```python
from build123d import *

# Parameters (mm, degrees)
F0_R     = 25.4
F0_R_2   = 15.875
F1_DEPTH = 8.89
F3_R     = 3.175
F4_REACH = 59.7812561211
F6_R     = 3.175
F7_REACH = 59.7812562211
F8_SIZE  = 0.762
F9_SIZE  = 0.762


with BuildPart() as f1:
    # F0 (on Right) → F1 (new body)
    with BuildSketch(Plane.YZ):
        Circle(F0_R)
        Circle(F0_R_2, mode=Mode.SUBTRACT)
    extrude(amount=F1_DEPTH)

    f4_end = f1.faces().sort_by_distance((4.445, -15.875, 0))[0]
    # F3 (on offset) → F4 (cut, up to a face of the model that its end follows)
    with BuildSketch(Plane.XZ.offset(25.4)):
        with Locations((4.064, 0)):
            Circle(F3_R)
    f4_long = extrude(amount=-F4_REACH, mode=Mode.PRIVATE)
    add(split(f4_long, bisect_by=f4_end, keep=Keep.ALL, mode=Mode.PRIVATE).solids().sort_by_distance((4.064, -25.4, 0))[0], mode=Mode.SUBTRACT)

    f7_end = f1.faces().sort_by_distance((0.457728864, -15.875, 0))[0]
    # F6 (on offset) → F7 (cut, up to a face of the model that its end follows)
    with BuildSketch(Plane.XY.offset(25.4)):
        with Locations((4.064, 0)):
            Circle(F6_R)
    f7_long = extrude(amount=-F7_REACH, mode=Mode.PRIVATE)
    add(split(f7_long, bisect_by=f7_end, keep=Keep.ALL, mode=Mode.PRIVATE).solids().sort_by_distance((4.064, 0, 25.4))[0], mode=Mode.SUBTRACT)

    # F8
    f8_edges = [f1.edges().sort_by_distance(p)[0] for p in [
        (0, -25.4, 0),
    ]]
    chamfer(f8_edges, length=F8_SIZE)

    # F9
    f9_edges = [f1.edges().sort_by_distance(p)[0] for p in [
        (8.89, -25.4, 0),
    ]]
    chamfer(f9_edges, length=F9_SIZE)


solid = f1.part
```
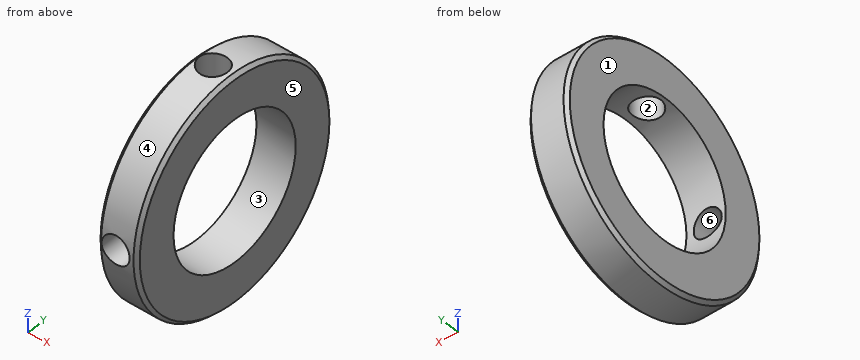
Input: part model. Units: mm. Frame: model coordinates. Face numbers are marked on the shaded views. A direction names the side the tool comes from. Give positions to 0.01 mm unless a question says otherwise; leave off trailing zeros. Order: outer loops, then holes, each group sorted by start corner. A loop starts at its lowest first (then second) coordinate and runs counter-clockwise, first axis right, second up. Notation, with made-up numbers: (-28.75, 28) - (-9.75, 28) arc R30 ccw to (-9.75, 66) - close; hole circle Ø10 at (26, 83.25). An arc over 180 degrees is marked (long way). One line per item, written item: value.
1. Cut plane C-C, the plane x = 5. Output: boundary loops of the cut face in (y, z) (3 decimals), and give its area (3 significant figures).
Determined:
outline: (-25.218, -3.034) arc R25.4 ccw (long way) to (3.034, 25.218) - (3.034, 15.582) arc R15.875 cw (long way) to (-15.582, -3.034) - close; (-25.218, 3.034) - (-15.582, 3.034) arc R15.875 cw to (-3.034, 15.582) - (-3.034, 25.218) arc R25.4 ccw to start
area: 1,120 mm2
2. Line query: probe 1 along X at (y, z) = (0, 19.5); probe 2 along Z at (x, y) = (6, -16); probe 3 along Z at (x, y) = (8, -5.5). Output: solid intervals per line, ascending.
Determined:
probe 1: 0 to 0.89, 7.24 to 8.89
probe 2: -19.73 to -2.52, 2.52 to 19.73
probe 3: -24.8 to -14.89, 14.89 to 24.8
3. Pin query (flat end, axial travel): pin 1 Ø5 at (x, y) = (4.5, -3) entering from +Z; pin 2 Ø4 at (x, z) = (4, 6.5) entering from -Y; pin 3 Ø5 at (x, y) = (4.064, 0) entering from -Z. Return the tip coordinate at first contact, or that it passes through.
Determined:
pin 1: z = 25.34
pin 2: y = -25
pin 3: z = -25.4
4. Cut plane A-A, the plane z = 0. Output: boundary loops of the cut face in (x, y) (3 decimals).
Determined:
outline: (0, -24.638) - (0.762, -25.4) - (0.889, -25.4) - (0.889, -15.875) - (0, -15.875) - close; (0, 15.875) - (8.89, 15.875) - (8.89, 24.638) - (8.128, 25.4) - (0.762, 25.4) - (0, 24.638) - close; (7.239, -25.4) - (8.128, -25.4) - (8.89, -24.638) - (8.89, -15.875) - (7.239, -15.875) - close
5. Cut plane B-B, the plane y = 0. Output: boundary loops of the cut face in (x, z) (3 decimals), and give its area (3 significant figures).
Determined:
outline: (0, -24.638) - (0.762, -25.4) - (8.128, -25.4) - (8.89, -24.638) - (8.89, -15.875) - (0, -15.875) - close; (0, 15.875) - (0.889, 15.875) - (0.889, 25.4) - (0.762, 25.4) - (0, 24.638) - close; (7.239, 15.875) - (8.89, 15.875) - (8.89, 24.638) - (8.128, 25.4) - (7.239, 25.4) - close
area: 108 mm2
6. Reachability of the marked faces 5 and 6 from +Z, -Z, +X, -X, +Y, -Y: full face, straight path, thin tool, end or side. Return the list, or none.
Determined:
face 5: +Z, -Z, +X, +Y, -Y
face 6: -Y
7. Draft query along Y for the marked faces 1, 2, 3 and 4. Return one class per face: released by +Y, released by -Y, zero draft, split by the parting line, or undercut.
Determined:
face 1: zero draft
face 2: undercut
face 3: undercut
face 4: split by the parting line
